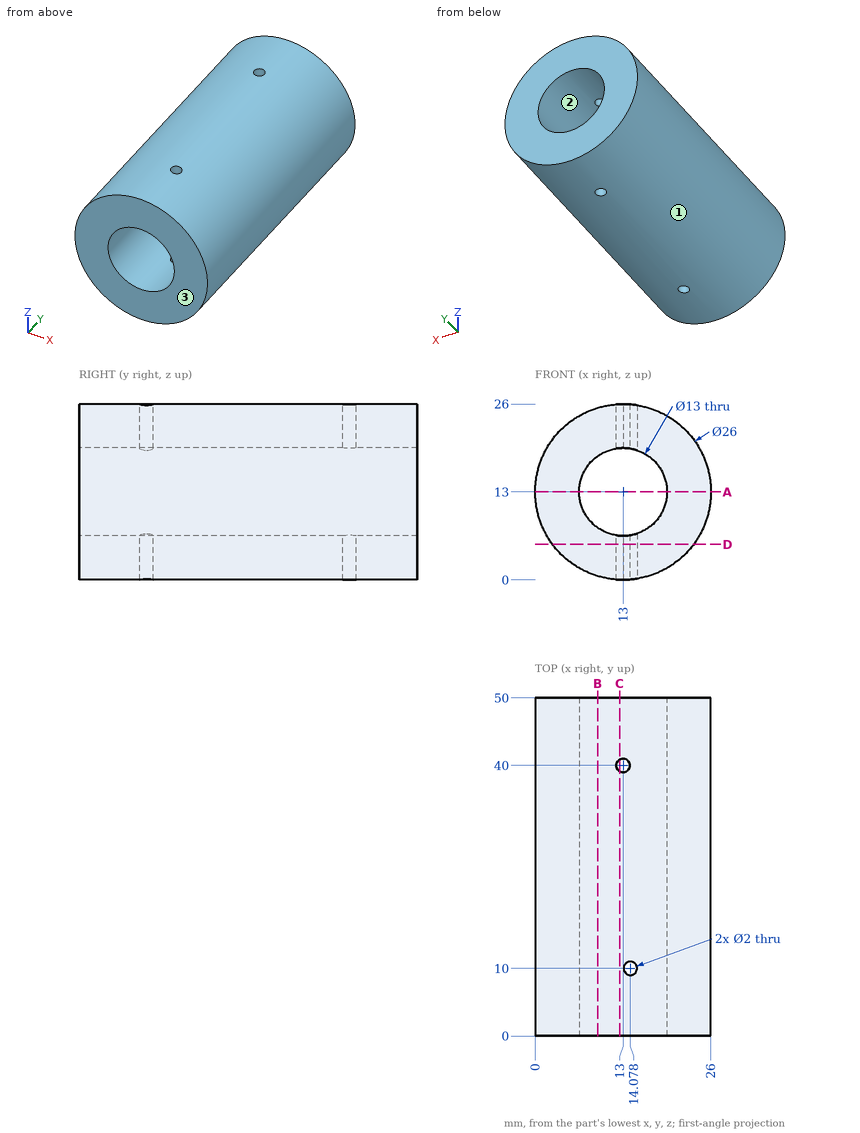
Verification items for this drawing (mm, ordinates from the low corner). Coordinates: 2 decimals unless noted, no trailing zeros. Write each loop counter-clockwise with the first axis right and the second up, starting at its lowest first coordinate (ties: lowest second). Pieces come first, ordered by that corner, then holes. Notation, with made-up numbers: M -12,86.25 L -8,86.25 A19 cw -8,92.25 Z; hole C 72,-30.75 d4. An arc over 180 degrees is marked long. One line per item, written item: value. Start each with the question number.
(1) Release check for a two-part mould opening along X. For the marked faces 1, 2 and 3 record: released by +X, released by -X, zero draft, split by the parting line, or undercut.
(2) Sectioned sample at A-A, the plane z = 13. Enter the section's corners in (x, y), and give its area (3 significant figures).
(3) Scan lines: line 1 along Y through (x, z) = (13, 23.5); line 2 along Z through (x, y) = (13, 20); line 3 along Z through (x, y) = (16.5, 39). Record each from-to range of solid material in increasing order. Write a range as [from, to].
(4) Sectioned sample at C-C, the plane x = 12.5. Enter the section's corners in (y, z).
(5) Sectioned sample at D-D, the plane z = 5.25. Enter the section's corners in (x, y).
(6) Depth check by flat-ended pin: pin 1 (1.8 mm diameter, centred on x = 13, y = 40, fed in from +Z); pin 2 (3 mm diameter, centred on y = 32.5, z = 11.5, fed in from -X); pin 3 (4 mm diameter, centred on x = 16, y = 14.5, fed in from -Z); pin 4 (12 mm diameter, centred on y = 29.5, z = 20, fed in from +X). Enter the tip coordinate at first touch or a pass-through.
(7) Sectioned sample at B-B, the plane x = 9.25. Enter the section's corners in (y, z).
Filled sheet:
1. face 1: split by the parting line
1. face 2: undercut
1. face 3: zero draft
2. outline: M 0,0 L 6.5,0 L 6.5,50 L 0,50 Z; M 19.5,0 L 26,0 L 26,50 L 19.5,50 Z
2. area: 650 mm²
3. line 1: [0, 39], [41, 50]
3. line 2: [0, 6.5], [19.5, 26]
3. line 3: [0.48, 7.52], [18.48, 25.52]
4. outline: M 0,0.01 L 39.13,0.01 L 39.13,6.52 L 0,6.52 Z; M 0,19.48 L 39.13,19.48 L 39.13,25.99 L 0,25.99 Z; M 40.87,0.01 L 50,0.01 L 50,6.52 L 40.87,6.52 Z; M 40.87,19.48 L 50,19.48 L 50,25.99 L 40.87,25.99 Z
5. outline: M 2.56,0 L 23.44,0 L 23.44,50 L 2.56,50 Z; hole C 13,40 d2; hole C 14.08,10 d2
6. pin 1: through
6. pin 2: x = 0
6. pin 3: z = 0.04
6. pin 4: x = 25.96
7. outline: M 0,0.55 L 50,0.55 L 50,7.69 L 0,7.69 Z; M 0,18.31 L 50,18.31 L 50,25.45 L 0,25.45 Z
